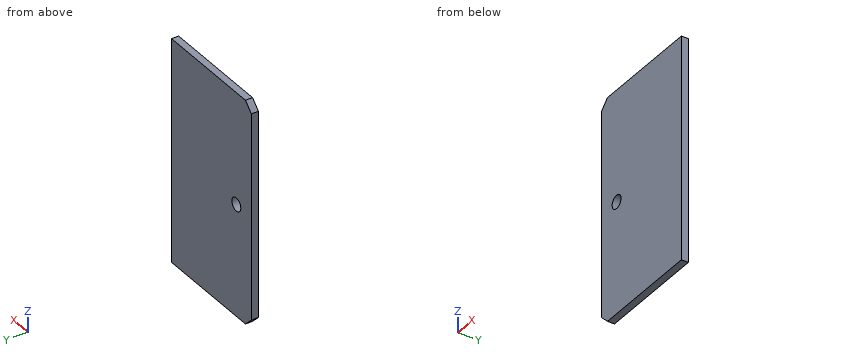
from build123d import *

# Parameters (mm, degrees)
SKETCH1_W           = 81.28
SKETCH1_H           = 50.8
BOSS_EXTRUDE1_DEPTH = 1.6002
SKETCH2_R           = 1.5
CUT_EXTRUDE1_DEPTH  = 1.6002
CHAMFER1_SIZE       = 2
CUT_EXTRUDE2_DEPTH  = 10


with BuildPart() as part:
    # Sketch1 → Boss-Extrude1 (new body)
    with BuildSketch(Plane(origin=(0, 0, 0), x_dir=(1, 0, 0), z_dir=(0, 1, 0))):
        Rectangle(SKETCH1_W, SKETCH1_H)
    extrude(amount=BOSS_EXTRUDE1_DEPTH)

    # Sketch2 → Cut-Extrude1 (cut)
    with BuildSketch(Plane(origin=(0, 1.6002, 0), x_dir=(1, 0, 0), z_dir=(0, 1, 0))):
        with Locations((-35.54, 0)):
            Circle(SKETCH2_R)
        with Locations((35.56, 0)):
            Circle(SKETCH2_R)
        Circle(SKETCH2_R)
    extrude(amount=-CUT_EXTRUDE1_DEPTH, mode=Mode.SUBTRACT)

    # Chamfer1
    chamfer1_edges = [part.edges().sort_by_distance(p)[0] for p in [
        (40.64, 0.8001, 25.4),
        (-40.64, 0.8001, 25.4),
        (-40.64, 0.8001, -25.4),
        (40.64, 0.8001, -25.4),
    ]]
    chamfer(chamfer1_edges, length=CHAMFER1_SIZE)

    # Sketch3 → Cut-Extrude2 (cut)
    with BuildSketch(Plane.XZ):
        Polygon((-13.546666667, 25.4), (-13.546666667, -25.4), (38.64, -25.4), (40.64, -23.4), (40.64, 23.4), (38.64, 25.4), align=None)
    extrude(amount=-CUT_EXTRUDE2_DEPTH, mode=Mode.SUBTRACT)


solid = part.part
Here's how the part is built. I have some questions about the finished solid (model axes, mm). Coordinates: 2 decimals unless noted, no trailing zeros. Order: outer loops, then holes, each group sorted by start corner. A loop starts at its lowest first (then second) coordinate and runs counter-clockwise, first axis right, second up. Notation, with made-up numbers: (-9.75, 24) -> (32.25, 24) arc R6 cw to (32.25, 32) -> close; hole circle Ø8 at (26, 12). An arc over 180 degrees is marked (long way). Answer in a Markdown table with one row per item.
(1) I want a section at A-A on z = 0. List the corners of the cut face in (x, y) for me.
Answer key:
| item | result |
|---|---|
| outline | (-40.64, 0) -> (-37.04, 0) -> (-37.04, 1.6) -> (-40.64, 1.6) -> close; (-34.04, 0) -> (-13.55, 0) -> (-13.55, 1.6) -> (-34.04, 1.6) -> close |
(2) I want a section at B-B on x = -35.54. List the corners of the cut face in (y, z) for me.
Answer key:
| item | result |
|---|---|
| outline | (0, -25.4) -> (1.6, -25.4) -> (1.6, -1.5) -> (0, -1.5) -> close; (0, 1.5) -> (1.6, 1.5) -> (1.6, 25.4) -> (0, 25.4) -> close |
(3) Please list where these lines run through material, in increasing order: probe 1 along Z at (x, y) = (-35.54, 1); probe 2 along X at (y, z) = (0.85, 0); probe 3 along Z at (x, y) = (-39, 0.3).
Answer key:
| item | result |
|---|---|
| probe 1 | -25.4 to -1.5, 1.5 to 25.4 |
| probe 2 | -40.64 to -37.04, -34.04 to -13.55 |
| probe 3 | -25.04 to 25.04 |
